CAD build for the part. Positions are in the model's coordinates, mm. Coordinates: 2 decimals unless noted, no trailing zeros. Loops run counter-clockwise (first coordinate to the right, second up) from the corner with the lowest first, then second, coordinate; pieces in that order, holes last. Notation, with made-up numbers: (24, 39.5) - (46, 39.5) arc R25 cw to (46, 78.5) - close; hole circle Ø9 at (-15, 85). An arc over 180 degrees is marked (long way). Put each result on its own line as item: value.
```python
from build123d import *

# Parameters (mm, degrees)
SKETCH1_W           = 95.25
SKETCH1_H           = 95.25
SKETCH1_R           = 3.175
SKETCH1_W_2         = 63.5
SKETCH1_H_2         = 63.5
BOSS_EXTRUDE1_DEPTH = 4


with BuildPart() as part:
    # Sketch1 → Boss-Extrude1 (new body)
    with BuildSketch(Plane(origin=(0, 0, 0), x_dir=(1, 0, 0), z_dir=(0, 1, 0))):
        Rectangle(SKETCH1_W, SKETCH1_H)
        with Locations((-38.1, 38.1)):
            Circle(SKETCH1_R, mode=Mode.SUBTRACT)
        with Locations((38.1, 38.1)):
            Circle(SKETCH1_R, mode=Mode.SUBTRACT)
        with Locations((38.1, -38.1)):
            Circle(SKETCH1_R, mode=Mode.SUBTRACT)
        with Locations((-38.1, -38.1)):
            Circle(SKETCH1_R, mode=Mode.SUBTRACT)
        Rectangle(SKETCH1_W_2, SKETCH1_H_2, mode=Mode.SUBTRACT)
    extrude(amount=BOSS_EXTRUDE1_DEPTH)


solid = part.part
```
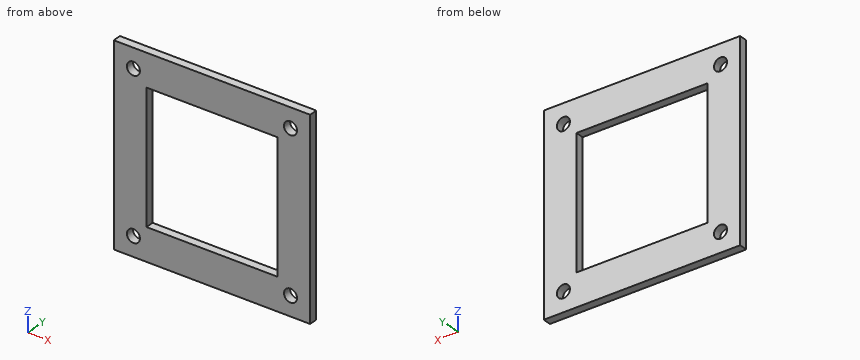
Q1. Slice it at B-B, the plane z = 38.1. Give the cut face in (x, y) (3 decimals).
Determined:
outline: (-47.625, 0) - (-41.275, 0) - (-41.275, 4) - (-47.625, 4) - close; (-34.925, 0) - (34.925, 0) - (34.925, 4) - (-34.925, 4) - close; (41.275, 0) - (47.625, 0) - (47.625, 4) - (41.275, 4) - close
Q2. Pin check, flat tip, straight feed: pin 1 Ø4 at (x, z) = (-38.1, -38.1) entering from -Y. Stop position of the tip, or through.
Determined:
pin 1: through
Q3. Slice it at C-C, the plane z = -14. Give the cut face in (x, y) (3 decimals).
Determined:
outline: (-47.625, 0) - (-31.75, 0) - (-31.75, 4) - (-47.625, 4) - close; (31.75, 0) - (47.625, 0) - (47.625, 4) - (31.75, 4) - close
Q4. Slice it at D-D, the plane x = -8. Give the cut face in (y, z) (3 decimals).
Determined:
outline: (0, -47.625) - (4, -47.625) - (4, -31.75) - (0, -31.75) - close; (0, 31.75) - (4, 31.75) - (4, 47.625) - (0, 47.625) - close
Q5. Wall check: L1, parallel to X at y = 1.4, z = 38.1 (3 decimals); L2, parallel to X at y = 2.75, z = -1 (3 decimals). Give the ranges that are in metal, low to high. Write a range as from..to.
Determined:
L1: -47.625..-41.275, -34.925..34.925, 41.275..47.625
L2: -47.625..-31.75, 31.75..47.625
Q6. Slice it at A-A, the plane x = 38.1. Give the cut face in (y, z) (3 decimals), then the cut area to 3 significant figures.
Determined:
outline: (0, -47.625) - (4, -47.625) - (4, -41.275) - (0, -41.275) - close; (0, -34.925) - (4, -34.925) - (4, 34.925) - (0, 34.925) - close; (0, 41.275) - (4, 41.275) - (4, 47.625) - (0, 47.625) - close
area: 330 mm2
